Source: CAD feature listing. Evaluate the final solid. Frame: model axes, mm. A direction names the side the tool comes from. Round coordinates to 2 decimals unless told otherwise and drop trailing zeros. Loops run counter-clockwise (first coordinate to the right, second up) from the corner with the lowest first, then second, coordinate; pieces in that order, holes last. Notation, with made-up numbers: (-33.75, 2.5) - (18.25, 2.5) arc R19 ccw to (18.25, 35.5) - close; hole circle Ø7 at (-10.5, 2). An arc over 180 degrees is marked (long way). One line per question, with ' | ' between items.
from build123d import *

# Parameters (mm, degrees)
SKETCH_1_W          = 45
SKETCH_1_H          = 45
EXTRUDE_1_DEPTH     = 100
FILLET_1_R          = 10
FILLET_2_R          = 0.5
SKETCH_2_R          = 5
CUT_EXTRUDE_1_DEPTH = 1
CUT_EXTRUDE_2_DEPTH = 12


with BuildPart() as part:
    # 草图1 → 凸台-拉伸1 (new body)
    with BuildSketch(Plane(origin=(0, 0, 0), x_dir=(1, 0, 0), z_dir=(0, 1, 0))):
        Rectangle(SKETCH_1_W, SKETCH_1_H)
    extrude(amount=-EXTRUDE_1_DEPTH)

    # 圆角1
    fillet_1_edges = [part.edges().sort_by_distance(p)[0] for p in [
        (22.5, -50, 22.5),
        (-22.5, -50, 22.5),
        (-22.5, -50, -22.5),
        (22.5, -50, -22.5),
    ]]
    fillet(fillet_1_edges, radius=FILLET_1_R)

    # 圆角2
    fillet_2_edges = [part.edges().sort_by_distance(p)[0] for p in [
        (0, 0, -22.5),
        (0, -100, -22.5),
        (22.5, 0, 0),
        (-22.5, 0, 0),
        (0, 0, 22.5),
        (-19.571067812, 0, 19.571067812),
        (19.571067812, 0, 19.571067812),
        (19.571067812, 0, -19.571067812),
        (-19.571067812, 0, -19.571067812),
        (-22.5, -100, 0),
        (22.5, -100, 0),
        (0, -100, 22.5),
        (-19.571067812, -100, 19.571067812),
        (19.571067812, -100, 19.571067812),
        (19.571067812, -100, -19.571067812),
        (-19.571067812, -100, -19.571067812),
    ]]
    fillet(fillet_2_edges, radius=FILLET_2_R)

    # 草图2 → 切除-拉伸1 (cut)
    with BuildSketch(Plane(origin=(0, 0, 0), x_dir=(1, 0, 0), z_dir=(0, 1, 0))):
        with Locations(Location((0, 0, 0), (0, 0, 270))):
            Circle(SKETCH_2_R)
    extrude(amount=-CUT_EXTRUDE_1_DEPTH, mode=Mode.SUBTRACT)

    # 草图3 → 切除-拉伸2 (cut)
    with BuildSketch(Plane(origin=(0, -1, 0), x_dir=(1, 0, 0), z_dir=(0, 1, 0))):
        Polygon((4.618802154, 0), (2.309401077, 4), (-2.309401077, 4), (-4.618802154, 0), (-2.309401077, -4), (2.309401077, -4), align=None)
    extrude(amount=-CUT_EXTRUDE_2_DEPTH, mode=Mode.SUBTRACT)


solid = part.part
1. Access query for faces 4 (the cylindrical face through (19.65, -50.69, -19.49)), 5 (the flat face through (4, -1, 2)). Directions: +Z, -Z, +X, -X, +Y, -Y. A direction counts if a zero-diameter tool reaches every point of the face in a straight line with its end or side. Return the directions, or none.
Worked out:
face 4: -Z, +X, +Y, -Y | face 5: +Y
2. Contact query for a flat-ended pin moving along its axis: P1, Ø4, axis at x = -2.5, z = 1, coming from the +Y side. Output: stop coordinate, or through.
Worked out:
P1: stops at y = -1
3. Section query C-C, the plane x = 0. Return loops of the section in (y, z).
Worked out:
outline: (-100, -22) arc R0.5 ccw to (-99.5, -22.5) - (-0.5, -22.5) arc R0.5 ccw to (0, -22) - (0, -5) - (-1, -5) - (-1, -4) - (-13, -4) - (-13, 4) - (-1, 4) - (-1, 5) - (0, 5) - (0, 22) arc R0.5 ccw to (-0.5, 22.5) - (-99.5, 22.5) arc R0.5 ccw to (-100, 22) - close
4. Material intervals for probe 1 along X at (y, z) = (-0.65, 0); probe 2 along Z at (x, y) = (1.5, -7); probe 3 along X at (y, z) = (-58.5, -18.5), sorted ascending.
Worked out:
probe 1: x = -22.5 to -5, 5 to 22.5 | probe 2: z = -22.5 to -4, 4 to 22.5 | probe 3: x = -20.5 to 20.5
5. Section query B-B, the plane y = -60.5. Return loops of the section in (x, z), plus the area to 3 significant figures.
Worked out:
outline: (-22.5, -12.5) arc R10 ccw to (-12.5, -22.5) - (12.5, -22.5) arc R10 ccw to (22.5, -12.5) - (22.5, 12.5) arc R10 ccw to (12.5, 22.5) - (-12.5, 22.5) arc R10 ccw to (-22.5, 12.5) - close | area: 1,940 mm2
6. Section query A-A, the plane y = -8. Return loops of the section in (x, z), plus the area to 3 significant figures.
Worked out:
outline: (-22.5, -12.5) arc R10 ccw to (-12.5, -22.5) - (12.5, -22.5) arc R10 ccw to (22.5, -12.5) - (22.5, 12.5) arc R10 ccw to (12.5, 22.5) - (-12.5, 22.5) arc R10 ccw to (-22.5, 12.5) - close; hole (-4.62, 0) - (-2.31, -4) - (2.31, -4) - (4.62, 0) - (2.31, 4) - (-2.31, 4) - close | area: 1,880 mm2
7. Mould query, pull axis Z, two halves, no side actions, for faces 1 (the flat face through (0, -7, -4)), 2 (the flat face through (22.5, -49, 0)), 3 (the cylindrical face through (-19.65, -50.69, 19.49)). Classes: released by +Z, released by -Z, zero draft, split by the parting line, or undercut.
Worked out:
face 1: undercut | face 2: zero draft | face 3: released by +Z
